Could you check a few things on this drawing? It's one solid part, dimensions in mm from its lowest x, y, z. A direction names the side the tool comes from. Give positions to 0.01 mm unless a question says otherwise; leave off trailing zeros. Loops run counter-clockwise (first coordinate to the right, second up) from the corner with the lowest first, then second, coordinate; pieces in that order, holes last. Notation, with made-up numbers: M 89.5,38.5 L 113.5,38.5 A30 cw 113.5,70.5 Z; hole C 11,0 d10. An arc over 180 degrees is marked long. Answer in a Markdown table with one row per item. Add a question column.
1. Thinking about a two-plate mould opening in Z: for the marked faces 1, 2, 3 and 4, which applies, released by +Z, released by -Z, zero draft, split by the parting line, or undercut?
2. If we section it at C-C on z = 14.25: List the corners of the cut face in (x, y) for me, then the cut area to 3 significant figures.
3. I'm going to push flat-ended pins straight in: pin 1 Ø1 at (y, z) = (19, 6.5) entering from -X; pin 2 Ø6 at (x, y) = (44, 5) entering from +Z; pin 3 Ø5.5 at (x, z) = (25, 15) entering from -Y; pin 4 Ø1.5 at (y, z) = (1.5, 12) entering from -X. Where does each tip first touch, or does it pass through?
4. I need wall thicknesses on line 1 along Y through (x, z) = (6, 2.4); line 2 along Z through (x, y) = (25, 2.65); line 3 along X through (y, z) = (5.5, 3). Which ranges of each line are inside material? Lowest first, please. Write a range as from..to.
5. If we section it at A-A on x = 13: List the corners of the cut face in (y, z) for me.
6. If we section it at D-D on x = 25: List the corners of the cut face in (y, z) for me, then the cut area to 3 significant figures.
7. Which directions (+Z, -Z, +X, -X, +Y, -Y) give clear straight access to the entire face, cutting with the end or side of a thin tool? Please do the marked faces 5, 6 and 7.
8. If we section it at B-B on y = 8: List the corners of the cut face in (x, z) for me, then the cut area to 3 significant figures.
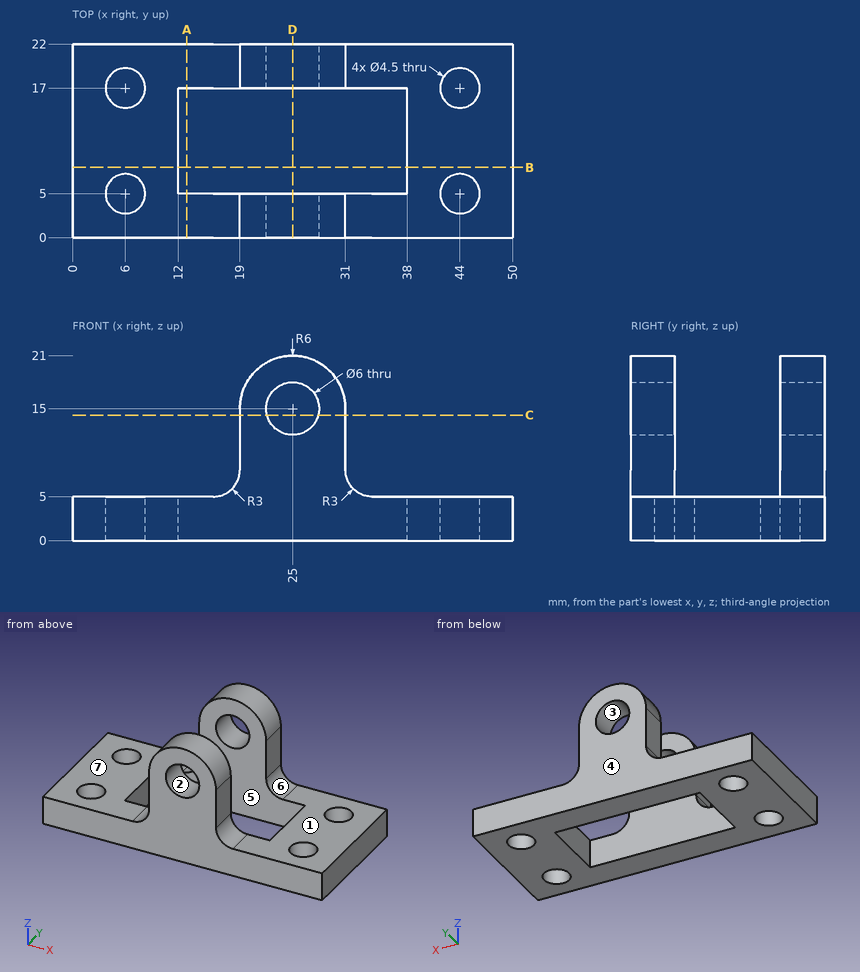
Results:
| question | item | result |
|---|---|---|
| 1 | face 1 | released by +Z |
| 1 | face 2 | undercut |
| 1 | face 3 | undercut |
| 1 | face 4 | zero draft |
| 2 | outline | M 19,0 L 22.1,0 L 22.1,5 L 19,5 Z; M 19,17 L 22.1,17 L 22.1,22 L 19,22 Z; M 27.9,0 L 31,0 L 31,5 L 27.9,5 Z; M 27.9,17 L 31,17 L 31,22 L 27.9,22 Z |
| 2 | area | 61.9 mm2 |
| 3 | pin 1 | x = 18.24 |
| 3 | pin 2 | z = 5 |
| 3 | pin 3 | through |
| 3 | pin 4 | x = 19 |
| 4 | line 1 | 0..2.75, 7.25..14.75, 19.25..22 |
| 4 | line 2 | 0..12, 18..21 |
| 4 | line 3 | 0..3.81, 8.19..12, 38..41.81, 46.19..50 |
| 5 | outline | M 0,0 L 5,0 L 5,5 L 0,5 Z; M 17,0 L 22,0 L 22,5 L 17,5 Z |
| 6 | outline | M 0,0 L 5,0 L 5,12 L 0,12 Z; M 0,18 L 5,18 L 5,21 L 0,21 Z; M 17,0 L 22,0 L 22,12 L 17,12 Z; M 17,18 L 22,18 L 22,21 L 17,21 Z |
| 6 | area | 150 mm2 |
| 7 | face 5 | +Z, -Z |
| 7 | face 6 | +Z, +X, +Y, -Y |
| 7 | face 7 | +Z, -X, +Y, -Y |
| 8 | outline | M 0,0 L 12,0 L 12,5 L 0,5 Z; M 38,0 L 50,0 L 50,5 L 38,5 Z |
| 8 | area | 120 mm2 |
